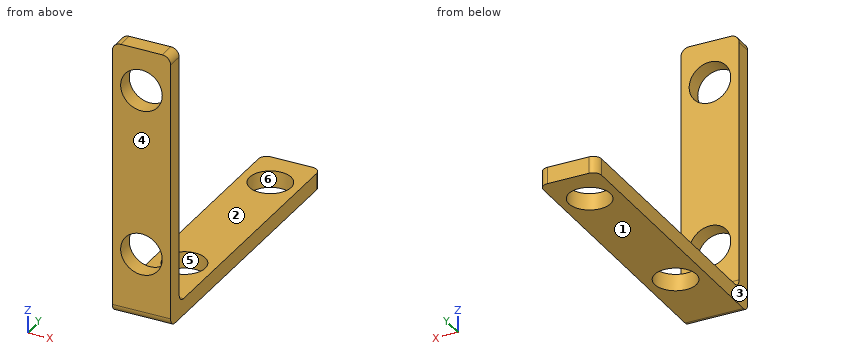
```python
from build123d import *

# Parameters (mm, degrees)
ESQUISSE1_W        = 7
ESQUISSE1_H        = 33
ESQUISSE1_R        = 2.5
BOSS_EXTRU_1_DEPTH = 2
ESQUISSE1_3_W      = 7
ESQUISSE1_3_H      = 2
BOSS_EXTRU_2_DEPTH = 33
CONG_2_DEPTH       = 7
CONG_2_2_OUTLINE_R = 2.5
CONG_2_2_DEPTH     = 2
CONG_2_START       = -1
CONG_2_3_DEPTH     = 4
CONG_2_4_DEPTH     = 9


with BuildPart() as part:
    # Esquisse1 → Boss.-Extru.1 (new body)
    with BuildSketch(Plane.XY):
        with Locations((3.5, 18.5)):
            Rectangle(ESQUISSE1_W, ESQUISSE1_H)
        with Locations((3.5, 10)):
            Circle(ESQUISSE1_R, mode=Mode.SUBTRACT)
        with Locations((3.5, 30)):
            Circle(ESQUISSE1_R, mode=Mode.SUBTRACT)
    extrude(amount=BOSS_EXTRU_1_DEPTH)

    # Esquisse1<3> → Boss.-Extru.2 (add)
    with BuildSketch(Plane.XY):
        with Locations((3.5, 1)):
            Rectangle(ESQUISSE1_3_W, ESQUISSE1_3_H)
    extrude(amount=BOSS_EXTRU_2_DEPTH)

    # Congé2: read off the stored shape, not the designer's step
    # Congé2 outline → Congé2 (add)
    with BuildSketch(Plane.YZ):
        with BuildLine():
            Line((2, 2), (3, 2))
            ThreePointArc((3, 2), (2.292893219, 2.292893219), (2, 3))
            Line((2, 3), (2, 2))
        make_face()
    extrude(amount=CONG_2_DEPTH)

    # Cong_2 2 outline → Cong_2 2 (cut)
    with BuildSketch(Plane(origin=(0, 0, 0), x_dir=(1, 0, 0), z_dir=(0, 1, 0))):
        with Locations((3.5, -8)):
            Circle(CONG_2_2_OUTLINE_R)
        with Locations((3.5, -28)):
            Circle(CONG_2_2_OUTLINE_R)
        with BuildLine():
            Line((7, -33), (7, -32))
            ThreePointArc((7, -32), (6.707106781, -32.707106781), (6, -33))
            Line((6, -33), (7, -33))
        make_face()
        with BuildLine():
            Line((0, -33), (1, -33))
            ThreePointArc((1, -33), (0.292893219, -32.707106781), (0, -32))
            Line((0, -32), (0, -33))
        make_face()
    extrude(amount=CONG_2_2_DEPTH, mode=Mode.SUBTRACT)

    # Cong_2 3 outline → Cong_2 3 (cut)
    with BuildSketch(Plane.XY.offset(CONG_2_START)):
        with BuildLine():
            ThreePointArc((0, 34), (0.292893219, 34.707106781), (1, 35))
            Line((1, 35), (0, 35))
            Line((0, 35), (0, 34))
        make_face()
        with BuildLine():
            ThreePointArc((6, 35), (6.707106781, 34.707106781), (7, 34))
            Line((7, 34), (7, 35))
            Line((7, 35), (6, 35))
        make_face()
    extrude(amount=CONG_2_3_DEPTH, mode=Mode.SUBTRACT)

    # Cong_2 4 outline → Cong_2 4 (cut)
    with BuildSketch(Plane.YZ.offset(CONG_2_START)):
        with BuildLine():
            ThreePointArc((1, 0), (0.292893219, 0.292893219), (0, 1))
            Line((0, 1), (0, 0))
            Line((0, 0), (1, 0))
        make_face()
    extrude(amount=CONG_2_4_DEPTH, mode=Mode.SUBTRACT)


solid = part.part
```
The model under review builds one solid part; all positions refer to its coordinate system, in mm. Face numbers are marked on the shaded views. A direction names the side the tool comes from. Coordinates: 2 decimals unless noted, no trailing zeros. Write each loop counter-clockwise with the first axis right and the second up, starting at its lowest first coordinate (ties: lowest second). Pieces come first, ordered by that corner, then holes. Notation, with made-up numbers: (59, 45.25) - (106, 45.25) arc R17 cw to (106, 50.25) - close; hole circle Ø2 at (-17, 35). An arc over 180 degrees is marked (long way). Answer in a Markdown table with one row per item. Add a question column.
Q1. For the marked faces 1 and 2, list the 3-axis set-ups (+Z, -Z, +X, -X, +Y, -Y) from which the entire face can be reached by the end or side of a thin tool; tool diameter is ignored.
Q2. Consider section A-A on z = 8. Give the boundary of the cut face in (x, y).
Q3. Draft analysis for pull direction Y (two halves, no side actions). For the marked faces 3, 4, 5 and 6, state which applies: +Y half, -Y half, draft (parallel to the pull), parting line (faces both ways), or undercut.
Q4. Consider section B-B on x = 5. Give the boundary of the cut face in (y, z), then the cut area to 3 significant figures.
Q5. Clearance check with flat-ended pins moving along their axes: pin 1 (1.5 mm diameter, centred on x = 2, z = 18, fed in from -Y); pin 2 (3.5 mm diameter, centred on x = 5, z = 10.5, fed in from +Y). State where each tip first meets the part, or that it passes through.
Q6. Consider section D-D on x = 2.25. Give the boundary of the cut face in (y, z), then the cut area to 3 significant figures.
Q7. To check wall thickness, follow line 1 along Y through (x, z) = (3.5, 1.2); line 2 along Z through (x, y) = (3.5, 1.1); line 3 along Y through (x, z) = (3.5, 0.6). State the ranges of each line that lie inside material, in increasing order. Write a range as from..to.
Answers below:
| question | item | result |
|---|---|---|
| 1 | face 1 | -Z, +X, -X, +Y, -Y |
| 1 | face 2 | +Z, +X, -X, +Y |
| 2 | outline | (0, 0) - (1, 0) - (1, 2) - (0, 2) - close; (6, 0) - (7, 0) - (7, 2) - (6, 2) - close |
| 3 | face 3 | draft |
| 3 | face 4 | -Y half |
| 3 | face 5 | undercut |
| 3 | face 6 | undercut |
| 4 | outline | (0, 1) arc R1 ccw to (1, 0) - (8, 0) - (8, 2) - (3, 2) arc R1 cw to (2, 3) - (2, 6) - (0, 6) - close; (0, 10) - (2, 10) - (2, 26) - (0, 26) - close; (0, 30) - (2, 30) - (2, 33) - (0, 33) - close; (12, 0) - (28, 0) - (28, 2) - (12, 2) - close; (32, 0) - (35, 0) - (35, 2) - (32, 2) - close |
| 4 | area | 100 mm² |
| 5 | pin 1 | y = 0 |
| 5 | pin 2 | y = 2 |
| 6 | outline | (0, 1) arc R1 ccw to (1, 0) - (7.83, 0) - (7.83, 2) - (3, 2) arc R1 cw to (2, 3) - (2, 5.83) - (0, 5.83) - close; (0, 10.17) - (2, 10.17) - (2, 25.83) - (0, 25.83) - close; (0, 30.17) - (2, 30.17) - (2, 33) - (0, 33) - close; (12.17, 0) - (27.83, 0) - (27.83, 2) - (12.17, 2) - close; (32.17, 0) - (35, 0) - (35, 2) - (32.17, 2) - close |
| 6 | area | 97.4 mm² |
| 7 | line 1 | 0..7.5, 12.5..27.5, 32.5..35 |
| 7 | line 2 | 0..5.5, 10.5..25.5, 30.5..33 |
| 7 | line 3 | 0.08..7.5, 12.5..27.5, 32.5..35 |
